Source: CAD feature listing. Evaluate the final solid. Frame: model axes, mm. A direction names the side the tool comes from. Give positions to 0.01 mm unless a question says otherwise; leave off trailing zeros. Order: outer loops, then holes, each group sorted by start corner. A loop starts at its lowest first (then second) coordinate and runs counter-clockwise, first axis right, second up. Notation, with made-up numbers: M -3,7.25 L 29,7.25 A13 ccw 29,29.25 Z; hole C 38.5,25.5 d1. An arc over 180 degrees is marked long. One line per question, with ' | ' between items. Start each with the question number.
Autodesk Inventor part; units mm, degrees
ref_plane "YZ Plane" through (0, 0, 0) normal (1, 0, 0) x (0, 1, 0)
ref_plane "XZ Plane" through (0, 0, 0) normal (0, 1, 0) x (-1, 0, 0)
ref_plane "XY Plane" through (0, 0, 0) normal (0, 0, 1) x (1, 0, 0)
sketch "Sketch1" plane through (0, 0, 0) normal (0, 1, 0) x (-1, 0, 0)
  line L0 (0, 0) -> (30, 0)
  line L1 (30, 0) -> (30, -30)
  line L2 (30, -30) -> (0, -30)
  line L3 (0, -30) -> (0, 0)
  line L4 (30, -15) -> (0, -15) construction
  line L5 (15, -30) -> (15, 0) construction
  line L6 (27.5, -2.5) -> (2.5, -2.5)
  line L7 (2.5, -2.5) -> (2.5, -27.5)
  line L8 (2.5, -27.5) -> (27.5, -27.5)
  line L9 (27.5, -27.5) -> (27.5, -2.5)
  dimension "d0" = 30
  dimension "d1" = 30
  dimension "d2" = 2.5
  dimension "d3" = 2.5
extrude "Extrusion1" add sketch "Sketch1" along normal blind 1000
sketch "Sketch2" plane through (0, 0, 0) normal (1, 0, 0) x (0, 0, -1)
  line L0 (30, 0) -> (0, 0) construction
  line L1 (30, 0) -> (30, 1000) construction
  line L2 (0, 1000) -> (30, 1000) construction
  line L3 (0, 0) -> (0, 1000) construction
  line L4 (0, 0) -> (0, 1000) construction
  line L5 (0, 125) -> (30, 125) construction
  line L6 (30, 0) -> (30, 1000) construction
  dimension "d6" = 125
sketch "Sketch3" plane through (-30, 0, -30) normal (-1, 0, 0) x (0, 0, 1)
  line L0 (30, 0) -> (0, 0) construction
  line L1 (30, 0) -> (30, 1000) construction
  line L2 (0, 1000) -> (30, 1000) construction
  line L3 (0, 0) -> (0, 1000) construction
  line L4 (30, 125) -> (0, 125) construction
  line L5 (30, 0) -> (30, 1000) construction
  line L6 (30, 875) -> (1.3146, 875) construction
  line L7 (0, 0) -> (0, 1000) construction
  dimension "d7" = 125
equation "\"d0\" = d1"
equation "\"d3\" = d2"
properties part number "1250mm_box_section" material "Steel, Mild"
Item 1: Pin query (flat end, axial travel): pin 1 Ø12 at (x, y) = (-24.5, 895) entering from +Z. Return the tip coordinate at first contact, or that it passes through.
Item 2: Cut plane C-C on x = -13.25. Return the cut outline in (y, z).
Item 3: Reachability of faces 1 (the flat face through (-2.5, 493, -15)), 2 (the flat face through (-28, 1000, -15)) from +Z, -Z, +X, -X, +Y, -Y: full face, straight path, thin tool, end or side. Return the list, or none.
Item 4: Line query: line 1 (X direction, y = 716, z = -3.5). Output: solid intervals per line, ascending.
Item 5: Cut plane A-A on z = -18.75. Return the cut outline in (x, y), and give its area (3 significant figures).
Item 6: Mould query, pull axis X, two halves, no side actions, for faces 3 (the flat face through (-15, 493, -30)), 4 (the flat face through (-15, 493, -27.5)), 5 (the flat face through (-30, 493, -15)). Classes: pulls with the +X half, pulls with the -X half, needs draft (parallel to the pull), parting line crosses it, or undercut.
Item 7: Cut plane B-B on y = 702. Return the cut outline in (x, z).
Results are:
1) pin 1: stops at z = 0
2) outline: M 0,-30 L 1000,-30 L 1000,-27.5 L 0,-27.5 Z; M 0,-2.5 L 1000,-2.5 L 1000,0 L 0,0 Z
3) face 1: +Y, -Y | face 2: +Z, -Z, +X, -X, +Y
4) line 1: x = -30 to -27.5, -2.5 to 0
5) outline: M -30,0 L -27.5,0 L -27.5,1000 L -30,1000 Z; M -2.5,0 L 0,0 L 0,1000 L -2.5,1000 Z | area: 5,000 mm2
6) face 3: needs draft | face 4: undercut | face 5: pulls with the -X half
7) outline: M -30,-30 L 0,-30 L 0,0 L -30,0 Z; hole M -27.5,-27.5 L -2.5,-27.5 L -2.5,-2.5 L -27.5,-2.5 Z
